Can you work these out from the model? Positions are in its coordinate system, mm. Face numbers are marked on the shaded views. A direction names the side the tool comes from. Give positions to 0.01 mm unless a question says otherwise; leave off trailing zeros. Order: outer loops, then holes, each group sorted by start corner. A loop starts at its lowest first (then second) coordinate and runs counter-clockwise, first axis right, second up. Notation, with made-up numbers: (36, -31) - (76, -31) arc R20 cw to (76, 0) - close; hole circle Ø9 at (50.5, 35.5). An arc over 180 degrees is marked (long way). Return JSON: item names as keys, results as strings.
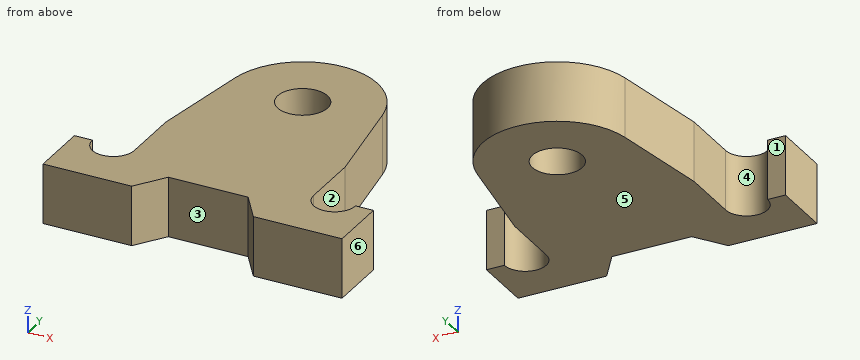
Autodesk Inventor part; units mm, degrees
ref_plane "YZ Plane" through (0, 0, 0) normal (1, 0, 0) x (0, 1, 0)
ref_plane "XZ Plane" through (0, 0, 0) normal (0, 1, 0) x (-1, 0, 0)
ref_plane "XY Plane" through (0, 0, 0) normal (0, 0, 1) x (1, 0, 0)
sketch "スケッチ1" plane through (0, 0, 0) normal (0, 0, 1) x (1, 0, 0)
  circle A0 centre (0, 0) radius 1.25
  circle A1 centre (0, 0) radius 3.75
  line L0 (-7.5, -10.5) -> (7.5, -10.5)
  line L1 (7.5, -10.5) -> (7.5, -7.5)
  line L2 (7.5, -7.5) -> (4.5, -7.5)
  line L3 (4.5, -7.5) -> (4.5, -4.5)
  line L4 (-7.5, -10.5) -> (-7.5, -7.5)
  line L5 (-7.5, -7.5) -> (-4.5, -7.5)
  line L6 (-4.5, -7.5) -> (-4.5, -4.5)
  line L7 (-4.5, -4.5) -> (-3.7049, 0.5799)
  line L8 (3.7049, 0.5799) -> (4.5, -4.5)
  arc A2 (-6.6, -7.5) -> (-4.5, -7.5) centre (-5.55, -7.5) ccw
  arc A3 (4.5, -7.5) -> (6.6, -7.5) centre (5.55, -7.5) ccw
  dimension "d0" = 2.5
  dimension "d1" = 7.5
  dimension "d2" = 15
  dimension "d3" = 3
  dimension "d4" = 3
  dimension "d5" = 3
  dimension "d6" = 3
  dimension "d7" = 3
  dimension "d8" = 3
  dimension "d9" = 4.5
  dimension "d10" = 7.5
  dimension "d11" = 2.1
  dimension "d12" = 2.1
extrude "押し出し1" add sketch "スケッチ1" along normal blind 3 contours A1 | A1 L8 L3 A3 L2 L1 L0 L4 L5 A2 L6 L7
sketch "スケッチ2" plane through (0, 0, 3) normal (0, 0, 1) x (1, 0, 0)
  circle A0 centre (0, 0) radius 1.25
  arc A1 (3.7049, 0.5799) -> (-3.7049, 0.5799) centre (0, 0) ccw
  line L0 (-3.7049, 0.5799) -> (-4.5, -4.5)
  line L1 (-4.5, -4.5) -> (-4.5, -7.5)
  arc A2 (-6.6, -7.5) -> (-4.5, -7.5) centre (-5.55, -7.5) ccw
  line L2 (-6.6, -7.5) -> (-7.5, -7.5)
  line L3 (-7.5, -7.5) -> (-7.5, -10.5)
  line L4 (-7.5, -10.5) -> (7.5, -10.5)
  line L5 (7.5, -10.5) -> (7.5, -7.5)
  line L6 (7.5, -7.5) -> (6.6, -7.5)
  arc A3 (4.5, -7.5) -> (6.6, -7.5) centre (5.55, -7.5) ccw
  line L7 (4.5, -7.5) -> (4.5, -4.5)
  line L8 (4.5, -4.5) -> (3.7049, 0.5799)
  line L9 (-3.0503, -10.5) -> (-2, -9)
  line L10 (-2, -9) -> (2, -9)
  line L11 (2, -9) -> (3.0503, -10.5)
  dimension "d15" = 125
  dimension "d16" = 125
  dimension "d17" = 4
  dimension "d18" = 2
  dimension "d19" = 1.5
extrude "押し出し2" cut sketch "スケッチ2" against normal blind 3 contours L4 L9 L10 L11
properties part number "新型４留め具" material "アルミニウム 2014-T4"
1. Suppose I cut it at C-C (z = 0.95). List the corners of the cut face in (x, y) for me.
Checks:
{"outline": "(-7.5, -10.5) - (-3.05, -10.5) - (-2, -9) - (2, -9) - (3.05, -10.5) - (7.5, -10.5) - (7.5, -7.5) - (6.6, -7.5) arc R1.05 cw to (4.5, -7.5) - (4.5, -4.5) - (3.7, 0.58) arc R3.75 ccw to (-3.7, 0.58) - (-4.5, -4.5) - (-4.5, -7.5) arc R1.05 cw to (-6.6, -7.5) - (-7.5, -7.5) - close; hole circle Ø2.5 at (0, 0)"}
2. On a 3-axis mill with a long thin cutter (end or side, diameter ignored), from which of +Z, -Z, +X, -X, +Y, -Y can I reach the whole of each face in a straight line? I mean the marked faces 1, 2 and 3. Say none if no direction works.
Checks:
{"face 1": "+Z, -Z, -X, +Y", "face 2": "+Z, -Z, +X, +Y", "face 3": "+Z, -Z, -Y"}
3. Suppose I cut it at A-A (x = 0). List the corners of the cut face in (y, z) for me.
Checks:
{"outline": "(-9, 0) - (-1.25, 0) - (-1.25, 3) - (-9, 3) - close; (1.25, 0) - (3.75, 0) - (3.75, 3) - (1.25, 3) - close"}
4. Thinking about a two-plate mould opening in X: for the marked faces 4, 5 and 6, which applies, +X half, -X half, draft (parallel to the pull), parting line (faces both ways), or undercut?
Checks:
{"face 4": "undercut", "face 5": "draft", "face 6": "+X half"}
5. For pin 1 Ø1.5 at (x, z) = (0, 1) entering from -Y; pin 2 Ø1 at (y, z) = (-3, 0.5) entering from +X; pin 3 Ø0.7 at (x, z) = (-7, 2) entering from +Y, each with a flat end and sliding along its axis, tell me the tip position at first contact or that it passes through.
Checks:
{"pin 1": "y = -9", "pin 2": "x = 4.34", "pin 3": "y = -7.5"}
6. Suppose I cut it at D-D (y = -8). List the corners of the cut face in (x, z) for me.
Checks:
{"outline": "(-7.5, 0) - (-6.47, 0) - (-6.47, 3) - (-7.5, 3) - close; (-4.63, 0) - (4.63, 0) - (4.63, 3) - (-4.63, 3) - close; (6.47, 0) - (7.5, 0) - (7.5, 3) - (6.47, 3) - close"}
7. Suppose I cut it at B-B (y = -9.5). List the corners of the cut face in (x, z) for me, plus the area to 3 significant figures.
Checks:
{"outline": "(-7.5, 0) - (-2.35, 0) - (-2.35, 3) - (-7.5, 3) - close; (2.35, 0) - (7.5, 0) - (7.5, 3) - (2.35, 3) - close", "area": "30.9 mm^2"}
8. If I drill on L1, parallel to Y at x = 0, z = 1.1; L2, parallel to X at y = -5, z = 0.95; L3, parallel to Y at x = -5.5, z = 1.35, over which ranges is the centre line in solid material (lowest first)? Write a range as [from, to].
Checks:
{"L1": "[-9, -1.25], [1.25, 3.75]", "L2": "[-4.5, 4.5]", "L3": "[-10.5, -8.55]"}
